Source: CAD feature listing. Evaluate the final solid. Frame: model axes, mm. A direction names the side the tool comes from. Coordinates: 2 decimals unless noted, no trailing zeros. Loops run counter-clockwise (first coordinate to the right, second up) from the corner with the lowest first, then second, coordinate; pieces in that order, holes last. Notation, with made-up numbers: (-15.5, -31.75) - (2.5, -31.75) arc R25 cw to (2.5, -0.75) - close; hole circle Ø10 at (16, -4). An arc over 180 degrees is marked (long way). Write item = value, one per line. Start each with the question number.
from build123d import *

# Parameters (mm, degrees)
SKETCH_1_W          = 55
SKETCH_1_H          = 38
EXTRUDE_1_DEPTH     = 3
SKETCH_2_R          = 1.5
CUT_EXTRUDE_1_DEPTH = 30
SKETCH_3_W          = 8
SKETCH_3_H          = 3
CUT_EXTRUDE_2_DEPTH = 30
SKETCH_5_W          = 12
SKETCH_5_H          = 3
CUT_EXTRUDE_4_DEPTH = 10
SKETCH_6_W          = 9
SKETCH_6_H          = 4
CUT_EXTRUDE_5_DEPTH = 10
SKETCH_7_R          = 0.5
CUT_EXTRUDE_6_DEPTH = 10


with BuildPart() as part:
    # 草图1 → 凸台-拉伸1 (new body)
    with BuildSketch(Plane.XY):
        Rectangle(SKETCH_1_W, SKETCH_1_H)
    extrude(amount=EXTRUDE_1_DEPTH)

    # 草图2 → 切除-拉伸1 (cut)
    with BuildSketch(Plane.XY.offset(3)):
        with Locations((16, 13.75)):
            Circle(SKETCH_2_R)
        with Locations((16, -13.75)):
            Circle(SKETCH_2_R)
        with Locations((-16, 13.75)):
            Circle(SKETCH_2_R)
        with Locations((-16, -13.75)):
            Circle(SKETCH_2_R)
    extrude(amount=-CUT_EXTRUDE_1_DEPTH, mode=Mode.SUBTRACT)

    # 草图3 → 切除-拉伸2 (cut)
    with BuildSketch(Plane.XY.offset(3)):
        with Locations((22, 17.5)):
            Rectangle(SKETCH_3_W, SKETCH_3_H)
        with Locations((22, -17.5)):
            Rectangle(SKETCH_3_W, SKETCH_3_H)
        with Locations((-22, 17.5)):
            Rectangle(SKETCH_3_W, SKETCH_3_H)
        with Locations((-22, -17.5)):
            Rectangle(SKETCH_3_W, SKETCH_3_H)
    extrude(amount=-CUT_EXTRUDE_2_DEPTH, mode=Mode.SUBTRACT)

    # 草图5 → 切除-拉伸4 (cut)
    with BuildSketch(Plane.XY.offset(3)):
        with Locations((0, -17.5)):
            Rectangle(SKETCH_5_W, SKETCH_5_H)
        with Locations((0, 17.5)):
            Rectangle(SKETCH_5_W, SKETCH_5_H)
    extrude(amount=-CUT_EXTRUDE_4_DEPTH, mode=Mode.SUBTRACT)

    # 草图6 → 切除-拉伸5 (cut)
    with BuildSketch(Plane(origin=(0, 0, 0), x_dir=(-1, 0, 0), z_dir=(0, 0, -1))):
        with Locations((-22, -8)):
            Rectangle(SKETCH_6_W, SKETCH_6_H)
        with Locations((-22, 0)):
            Rectangle(SKETCH_6_W, SKETCH_6_H)
        with Locations((-22, 8)):
            Rectangle(SKETCH_6_W, SKETCH_6_H)
        with Locations((22, -8)):
            Rectangle(SKETCH_6_W, SKETCH_6_H)
        with Locations((22, 0)):
            Rectangle(SKETCH_6_W, SKETCH_6_H)
        with Locations((22, 8)):
            Rectangle(SKETCH_6_W, SKETCH_6_H)
    extrude(amount=-CUT_EXTRUDE_5_DEPTH, mode=Mode.SUBTRACT)

    # 草图7 → 切除-拉伸6 (cut)
    with BuildSketch(Plane(origin=(0, 0, 0), x_dir=(-1, 0, 0), z_dir=(0, 0, -1))):
        with Locations((-18.212132034, -16.212132034)):
            Circle(SKETCH_7_R)
        with Locations((-25.787867966, -16.212132034)):
            Circle(SKETCH_7_R)
        with Locations((-25.787867966, 16.212132034)):
            Circle(SKETCH_7_R)
        with Locations((-18.212132034, 16.212132034)):
            Circle(SKETCH_7_R)
        with Locations((-5.787867966, -16.212132034)):
            Circle(SKETCH_7_R)
        with Locations((25.787867966, -16.212132034)):
            Circle(SKETCH_7_R)
        with Locations((18.212132034, -16.212132034)):
            Circle(SKETCH_7_R)
        with Locations((18.212132034, 16.212132034)):
            Circle(SKETCH_7_R)
        with Locations((25.787867966, 16.212132034)):
            Circle(SKETCH_7_R)
        with Locations((-5.787867966, 16.212132034)):
            Circle(SKETCH_7_R)
        with Locations((5.787867966, 16.212132034)):
            Circle(SKETCH_7_R)
        with Locations((5.787867966, -16.212132034)):
            Circle(SKETCH_7_R)
    extrude(amount=-CUT_EXTRUDE_6_DEPTH, mode=Mode.SUBTRACT)


solid = part.part
Item 1: Cut plane B-B (y = -13.75). Return the cut outline in (x, z), then the cut area to 3 significant figures.
Item 2: Cut plane C-C (x = -16). Return the cut outline in (y, z).
Item 3: First-contact query: pin 1 (4 mm diameter, centred on x = -16, y = -13.75, fed in from -Z); pin 2 (0.9 mm diameter, centred on x = -23.5, z = 1, fed in from -Y); pin 3 (0.9 mm diameter, centred on x = 23, z = 1.5, fed in from +Y). Flat tips, straight axial feed; report the tip coordinate or a pass-through.
Item 4: Cut plane A-A (x = -23). Return the cut outline in (y, z).
Item 5: Material intervals for L1, parallel to Y at x = -16, z = 2.15; L2, parallel to Y at x = 24, z = 0.35; L3, parallel to X at y = 8, z = 2.95, sorted ascending. Write a range as [from, to].
Item 6: Reachability of faces 4 (the flat face through (26.5, -8, 1)), 5 (the flat face through (-18, 18, 2)) from +Z, -Z, +X, -X, +Y, -Y: full face, straight path, thin tool, end or side. Return the list, or none.
Item 7: Cut plane D-D (z = 0.5). State how many separate pieces and enclosed holes the cut face has, then the cut area to 3 significant figures.
Item 8: Draft query along Y for faces 1 (the flat face through (-18, -18, 2)), 2 (the cylindrical face through (-17.5, 13.8, 1.5)), 3 (the flat face through (27, 19, 1)). Return one class per face: released by +Y, released by -Y, zero draft, split by the parting line, or undercut.
Responses:
q1.outline = (-27.5, 0) - (-17.5, 0) - (-17.5, 3) - (-27.5, 3) - close; (-14.5, 0) - (14.5, 0) - (14.5, 3) - (-14.5, 3) - close; (17.5, 0) - (27.5, 0) - (27.5, 3) - (17.5, 3) - close
q1.area = 147 mm2
q2.outline = (-19, 0) - (-15.25, 0) - (-15.25, 3) - (-19, 3) - close; (-12.25, 0) - (12.25, 0) - (12.25, 3) - (-12.25, 3) - close; (15.25, 0) - (19, 0) - (19, 3) - (15.25, 3) - close
q3.pin_1 = 0
q3.pin_2 = -16
q3.pin_3 = 16
q4.outline = (-16, 0) - (-10, 0) - (-10, 3) - (-16, 3) - close; (-6, 0) - (-2, 0) - (-2, 3) - (-6, 3) - close; (2, 0) - (6, 0) - (6, 3) - (2, 3) - close; (10, 0) - (16, 0) - (16, 3) - (10, 3) - close
q5.L1 = [-19, -15.25], [-12.25, 12.25], [15.25, 19]
q5.L2 = [-16, -10], [-6, -2], [2, 6], [10, 16]
q5.L3 = [-27.5, -26.5], [-17.5, 17.5], [26.5, 27.5]
q6.face_4 = +Z, -Z
q6.face_5 = +Z, -Z, +Y
q7.separate_pieces = 1
q7.enclosed_holes = 10
q7.area = 1,670 mm2
q8.face_1 = zero draft
q8.face_2 = undercut
q8.face_3 = released by +Y
